from build123d import *
from build123d.topology import SkipClean

# Parameters (mm, degrees)
SKETCH1_R           = 15
BOSS_EXTRUDE1_DEPTH = 70


with BuildPart() as part:
    # Sketch1 → Boss-Extrude1 (new body)
    with BuildSketch(Plane(origin=(0, 110.196823778, 0), x_dir=(1, 0, 0), z_dir=(0, 1, 0))):
        with Locations(Location((110.196823778, -15, 0), (0, 0, 270))):
            Circle(SKETCH1_R)
    extrude(amount=BOSS_EXTRUDE1_DEPTH)

    # Sketch2 → Revolve1 (revolve)
    with SkipClean():  # the faces are left unmerged after this step: merging them gives an invalid solid
        with BuildSketch(Plane(origin=(110.196823778, 0, 0), x_dir=(0, 0, -1), z_dir=(1, 0, 0))):
            with BuildLine():
                ThreePointArc((-30, 180.196823778), (-15, 165.196823778), (0, 180.196823778))
                Line((0, 180.196823778), (-30, 180.196823778))
            make_face()
            with BuildLine():
                Line((-30, 180.196823778), (0, 180.196823778))
                ThreePointArc((0, 180.196823778), (-15, 195.196823778), (-30, 180.196823778))
            make_face()
        revolve(axis=Axis((110.196823778, 180.196823778, 0), (0, 0, 1)))

    # Sketch2_3 → Revolve2 (revolve)
    with SkipClean():  # the faces are left unmerged after this step: merging them gives an invalid solid
        with BuildSketch(Plane(origin=(110.196823778, 0, 0), x_dir=(0, 0, -1), z_dir=(1, 0, 0))):
            with BuildLine():
                ThreePointArc((0, 110.196823778), (-15, 125.196823778), (-30, 110.196823778))
                Line((-30, 110.196823778), (0, 110.196823778))
            make_face()
            with BuildLine():
                Line((0, 110.196823778), (-30, 110.196823778))
                ThreePointArc((-30, 110.196823778), (-15, 95.196823778), (0, 110.196823778))
            make_face()
        revolve(axis=Axis((110.196823778, 110.196823778, 30), (0, 0, -1)))


solid = part.part
Work out the finished part from the listing and answer in its coordinate system (mm). Round coordinates to 2 decimals unless told otherwise and drop trailing zeros. Write each loop counter-clockwise with the first axis right and the second up, starting at its lowest first coordinate (ties: lowest second). Pieces come first, ordered by that corner, then holes. Notation, with made-up numbers: (2.25, 16.25) -> (44.25, 16.25) arc R16 ccw to (44.25, 40.25) -> close; hole circle Ø7 at (-3, 3). An arc over 180 degrees is marked (long way). Answer as CSV lines item,"result". Start each with the question number.
(1) The part is cut by section C-C, the plane y = 135.5. Give the vertices of the cut face in (x, z).
(2) Each of these flat-tipped pins is pushed along its axis until it touches: pin 1 (1.5 mm diameter, centred on x = 108.5, y = 171.5, fed in from +Z); pin 2 (4 mm diameter, centred on x = 115.5, z = 25.5, fed in from +Y); pin 3 (5 mm diameter, centred on x = 116.5, y = 114.5, fed in from -Z). Where does it stop, or does it pass through?
(3) The part is cut by section D-D, the plane y = 186. Give the vertices of the cut face in (x, z), then the cut area to 3 significant figures.
(4) Find the intervals of material crossed by probe 1 along X at (y, z) = (132.5, 15); probe 2 along Z at (x, y) = (122.25, 169.5); probe 3 along Z at (x, y) = (101.25, 151), in increasing order.
(5) The part is cut by section A-A, the plane z = 15. Give the vertices of the cut face in (x, y), then the cut area to 3 significant figures.
(6) The part is cut by section B-B, the plane x = 108.25. Give the vertices of the cut face in (y, z), then the cut area to 3 significant figures.
Output values:
1,outline,"circle Ø30 at (110.2, 15)"
2,pin 1,"stops at z = 29.97"
2,pin 2,"stops at y = 191.58"
2,pin 3,"stops at z = 0.49"
3,outline,"circle Ø27.66 at (110.2, 15)"
3,area,"601 mm²"
4,probe 1,"x = 95.2 to 125.2"
4,probe 2,"z = 6.07 to 23.93"
4,probe 3,"z = 2.96 to 27.04"
5,outline,"(95.2, 110.2) arc R15 ccw to (125.2, 110.2) -> (125.2, 180.2) arc R15 ccw to (95.2, 180.2) -> close"
5,area,"2,810 mm²"
6,outline,"(110.2, 0.13) -> (180.2, 0.13) arc R14.87 ccw to (180.2, 29.87) -> (110.2, 29.87) arc R14.87 ccw to start"
6,area,"2,780 mm²"
